```python
from build123d import *

# Parameters (mm, degrees)
F1_DEPTH = 38.1
F2_R     = 15.340009
F3_DEPTH = 38.1


with BuildPart() as f1:
    # F0 (on Front) → F1 (new body)
    with BuildSketch(Plane.XZ):
        Polygon((10.681883, 0.728829), (4.709757, 9.615196), (-5.972126, 8.886367), (-10.681883, -0.728829), (-4.709757, -9.615196), (5.972126, -8.886367), align=None)
    extrude(amount=F1_DEPTH)

    # F2 (on Front) → F3 (join)
    with BuildSketch(Plane.XZ):
        Circle(F2_R)
    extrude(amount=-F3_DEPTH)


solid = f1.part
```
Design review of the part built by this model. Coordinates are the model's own, in mm. A direction names the side the tool comes from. Round coordinates to 2 decimals unless told otherwise and drop trailing zeros. Order: outer loops, then holes, each group sorted by start corner. A loop starts at its lowest first (then second) coordinate and runs counter-clockwise, first axis right, second up. Notation, with made-up numbers: M 87,41 L 101,41 A24 ccw 101,73 Z; hole C 84,7 d2. An arc over 180 degrees is marked long. Put each result on its own line as item: value.
Q1. Consider section D-D (z = -12.5). State the section outline as (x, y) points, and give its area (3 significant figures).
Reported:
outline: M -8.89,0 L 8.89,0 L 8.89,38.1 L -8.89,38.1 Z
area: 678 mm²
Q2. Consider section A-A (y = -17.5). State the section outline as (x, z) points.
Reported:
outline: M -10.68,-0.73 L -4.71,-9.62 L 5.97,-8.89 L 10.68,0.73 L 4.71,9.62 L -5.97,8.89 Z
Q3. Insertion check: pin 1 Ø1 at (x, y) = (-6.5, -9.5) entering from -Z; pin 2 Ø6 at (x, y) = (9.5, 29.5) entering from -Z; pin 3 Ø4 at (y, z) = (12.5, 8.5) entering from -X. Each pin has a flat end and moves straight along its axis. Give the tip position at first contact, or say it passes through.
Reported:
pin 1: z = -7.7
pin 2: z = -13.89
pin 3: x = -13.89
Q4. Machinability: for faces 1 (the face through (-7.738, -18.783, -5.11)), 2 (the face through (-0.556, -18.783, 9.256)), 3 (the face through (-7, 0, -7)), 4 (the face through (0.556, -18.783, -9.256)), which of the approach directions +Z, -Z, +X, -X, +Y, -Y give a long, thin tool a straight path to every point of the face, cutting with its end or side? Answer none if there is none.
Reported:
face 1: -Z, -X, -Y
face 2: +Z, -X, -Y
face 3: -Y
face 4: -Z, +X, -Y
Q5. Consider section C-C (x = 0.5). State the section outline as (y, z) points.
Reported:
outline: M -38.1,-9.26 L 0,-9.26 L 0,-15.33 L 38.1,-15.33 L 38.1,15.33 L 0,15.33 L 0,9.33 L -38.1,9.33 Z
Q6. To check wall thickness, follow line 1 (Y direction, x = 6.5, z = -12); line 2 (X direction, y = 12, z = 12.5); line 3 (X direction, y = -6.5, z = -4). State the ranges of each line that lie inside material, in increasing order.
Reported:
line 1: 0 to 38.1
line 2: -8.89 to 8.89
line 3: -8.48 to 8.37
Q7. Consider section B-B (z = 4). State the section outline as (x, y) points, and give its area (3 significant figures).
Reported:
outline: M -14.81,0 L -8.37,0 L -8.37,-38.1 L 8.48,-38.1 L 8.48,0 L 14.81,0 L 14.81,38.1 L -14.81,38.1 Z
area: 1,770 mm²
